```python
from build123d import *

# Parameters (mm, degrees)
SKETCH_3_R          = 18
EXTRUDE_1_DEPTH     = 50
FILLET_2_R          = 2
SKETCH_4_R          = 6.5
EXTRUDE_2_DEPTH     = 3
SKETCH_5_R          = 18
EXTRUDE_3_DEPTH     = 32.5
SKETCH_6_R          = 11
EXTRUDE_4_DEPTH     = 2.3
SKETCH_7_R          = 4
EXTRUDE_5_DEPTH     = 17
CUT_EXTRUDE_START   = -15
CUT_EXTRUDE_1_DEPTH = 15
SKETCH_10_R         = 1.5
CUT_EXTRUDE_2_DEPTH = 8
SKETCH_11_R         = 1.585
EXTRUDE_6_DEPTH     = 2
SKETCH_14_R         = 1.5
CUT_EXTRUDE_3_DEPTH = 7


with BuildPart() as part:
    # 草图3 → 凸台-拉伸1 (new body)
    with BuildSketch(Plane(origin=(0, 0, 0), x_dir=(1, 0, 0), z_dir=(0, 1, 0))):
        with Locations(Location((0, 0, 0), (0, 0, 270))):
            Circle(SKETCH_3_R)
    extrude(amount=EXTRUDE_1_DEPTH)

    # 圆角2
    fillet_2_edges = [part.edges().sort_by_distance(p)[0] for p in [
        (0, 50, -18),
    ]]
    fillet(fillet_2_edges, radius=FILLET_2_R)

    # 草图4 → 凸台-拉伸2 (add)
    with BuildSketch(Plane.XZ):
        with Locations(Location((0, 0, 0), (0, 0, 270))):
            Circle(SKETCH_4_R)
    extrude(amount=EXTRUDE_2_DEPTH)

    # 草图5 → 凸台-拉伸3 (add)
    with BuildSketch(Plane(origin=(0, 50, 0), x_dir=(1, 0, 0), z_dir=(0, 1, 0))):
        with Locations(Location((0, 0, 0), (0, 0, 270))):
            Circle(SKETCH_5_R)
    extrude(amount=EXTRUDE_3_DEPTH)

    # 草图6 → 凸台-拉伸4 (add)
    with BuildSketch(Plane(origin=(0, 82.5, 0), x_dir=(1, 0, 0), z_dir=(0, 1, 0))):
        with Locations(Location((0, 0, 0), (0, 0, 270))):
            Circle(SKETCH_6_R)
    extrude(amount=EXTRUDE_4_DEPTH)

    # 草图7 → 凸台-拉伸5 (add)
    with BuildSketch(Plane(origin=(0, 84.8, 0), x_dir=(1, 0, 0), z_dir=(0, 1, 0))):
        with Locations(Location((0, 0, 0), (0, 0, 270))):
            Circle(SKETCH_7_R)
    extrude(amount=EXTRUDE_5_DEPTH)

    # 草图8 → 切除-拉伸1 (cut)
    with BuildSketch(Plane(origin=(0, 101.8, 0), x_dir=(1, 0, 0), z_dir=(0, 1, 0)).offset(CUT_EXTRUDE_START)):
        with BuildLine():
            Line((3, 2.645751311), (3, -2.645751311))
            ThreePointArc((3, -2.645751311), (4, 0), (3, 2.645751311))
        make_face()
    extrude(amount=CUT_EXTRUDE_1_DEPTH, mode=Mode.SUBTRACT)

    # 草图10 → 切除-拉伸2 (cut)
    with BuildSketch(Plane(origin=(0, 82.5, 0), x_dir=(1, 0, 0), z_dir=(0, 1, 0))):
        with Locations(Location((-9.899494937, 9.899494937, 0), (0, 0, 270))):
            Circle(SKETCH_10_R)
        with Locations(Location((9.899494937, 9.899494937, 0), (0, 0, 90))):
            Circle(SKETCH_10_R)
        with Locations(Location((9.899494937, -9.899494937, 0), (0, 0, 270))):
            Circle(SKETCH_10_R)
        with Locations(Location((-9.899494937, -9.899494937, 0), (0, 0, 90))):
            Circle(SKETCH_10_R)
    extrude(amount=-CUT_EXTRUDE_2_DEPTH, mode=Mode.SUBTRACT)

    # 草图11 → 凸台-拉伸6 (add)
    with BuildSketch(Plane.XZ.offset(3)):
        with Locations(Location((0, 0, 0), (0, 0, 270))):
            Circle(SKETCH_11_R)
    extrude(amount=EXTRUDE_6_DEPTH)

    # 草图14 → 切除-拉伸3 (cut)
    with BuildSketch(Plane(origin=(3, 0, 0), x_dir=(0, 0, -1), z_dir=(1, 0, 0))):
        with Locations((0, 97.8)):
            Circle(SKETCH_14_R)
    extrude(amount=-CUT_EXTRUDE_3_DEPTH, mode=Mode.SUBTRACT)


solid = part.part
```
Read the model definition and answer for the solid it produces. Units are mm, in the model's axes. A direction names the side the tool comes from. Give positions to 0.01 mm unless a question says otherwise; leave off trailing zeros. Loops run counter-clockwise (first coordinate to the right, second up) from the corner with the lowest first, then second, coordinate; pieces in that order, holes last.
Item 1: For faces 1 (the flat face through (0, 101.8, 0)), 2 (the flat face through (-1.4, -3, -1.4)), 3 (the cylindrical face through (5.407, 23.664, 17.169)), 4 (the flat face through (3, 94, 0)), 5 (the cylindrical face through (-3.905, 93.181, -0.867)), determine the directions among +Z, -Z, +X, -X, +Y, -Y from which every point of the face is accessible in a straight line to the end or side of a thin tool.
Item 2: The part is cut by section B-B (y = 77). Write down the section's boundary in (x, z), and give its area (3 significant figures).
Item 3: The part is cut by section A-A (x = 0). Write down the section's boundary in (y, z) (3 decimals).
Item 4: Find the intervals of material crossed by line 1 along Y through (x, z) = (1, 0); line 2 along Y through (x, z) = (5.5, 9); line 3 along Y through (x, z) = (-13, 3), in increasing order.
Item 5: The part is cut by section C-C (y = 97.8). Write down the section's boundary in (x, z), and give its area (3 significant figures).
Item 6: Each of these flat-tipped pins is pushed along its axis until it touches: pin 1 Ø3.5 at (y, z) = (97.8, 0) entering from +X; pin 2 Ø3 at (y, z) = (44, 9) entering from -X; pin 3 Ø3 at (y, z) = (65.5, 6.5) entering from +X. Where does it stop, or does it pass through?
Item 7: The part is cut by section D-D (y = 17). Write down the section's boundary in (x, z).
Taken from the geometry:
1. face 1: +Z, -Z, +X, -X, +Y
1. face 2: -Y
1. face 3: +Y, -Y
1. face 4: +Z, -Z, +X, +Y
1. face 5: +Y
2. outline: circle Ø36 at (0, 0); hole circle Ø3 at (-9.9, -9.9); hole circle Ø3 at (-9.9, 9.9); hole circle Ø3 at (9.9, -9.9); hole circle Ø3 at (9.9, 9.9)
2. area: 990 mm2
3. outline: (-5, -1.585) - (-3, -1.585) - (-3, -6.5) - (0, -6.5) - (0, -18) - (48, -18) arc R2 ccw to (50, -16) - (50, -18) - (82.5, -18) - (82.5, -11) - (84.8, -11) - (84.8, -4) - (101.8, -4) - (101.8, 4) - (84.8, 4) - (84.8, 11) - (82.5, 11) - (82.5, 18) - (50, 18) - (50, 16) arc R2 ccw to (48, 18) - (0, 18) - (0, 6.5) - (-3, 6.5) - (-3, 1.585) - (-5, 1.585) - close; hole circle Ø3 at (97.8, 0)
4. line 1: y = -5 to 96.3, 99.3 to 101.8
4. line 2: y = 0 to 84.8
4. line 3: y = 0 to 82.5
5. outline: (-3.71, -1.5) arc R4 ccw to (3, -2.65) - (3, -1.5) - close; (-3.71, 1.5) - (3, 1.5) - (3, 2.65) arc R4 ccw to start
5. area: 25.9 mm2
6. pin 1: stops at x = 3
6. pin 2: stops at x = -16.36
6. pin 3: stops at x = 17.29
7. outline: circle Ø36 at (0, 0)
